Geometry check sheet. Reference: drawing and pictorial views, mm from the part's lowest x, y, z. Give positions to 0.01 mm unless a question says otherwise; leave off trailing zeros. Order: outer loops, then holes, each group sorted by start corner. A loop starts at its lowest first (then second) coordinate and runs counter-clockwise, first axis right, second up.
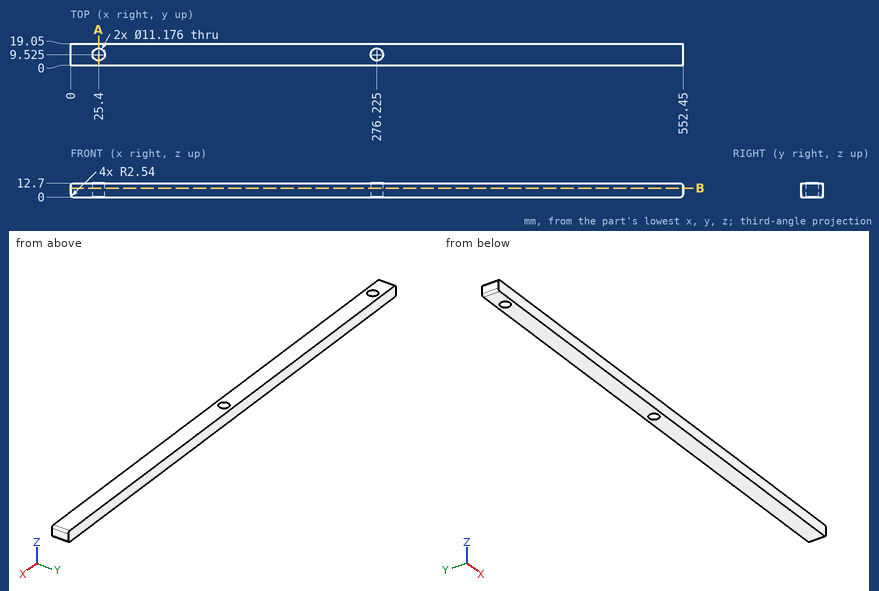
(1) Gauge pin test, flat end, axial feed: pin 1 Ø9 at (x, y) = (25.4, 9.525) entering from -Z. Record the tip position at first contact, or that the pin passes through.
Response values:
pin 1: passes through
(2) Cross-section at B-B on z = 8.25. Enter the section's corners in (x, y) (3 decimals), then the cut area to 3 significant figures.
Response values:
outline: (0, 0) - (552.45, 0) - (552.45, 19.05) - (0, 19.05) - close; hole circle Ø11.176 at (25.4, 9.525); hole circle Ø11.176 at (276.225, 9.525)
area: 10,300 mm2
(3) Cross-section at A-A on x = 25.4. Enter the section's corners in (y, z), then the cut area to 4 significant figures.
Response values:
outline: (0, 0) - (3.94, 0) - (3.94, 12.7) - (0, 12.7) - close; (15.11, 0) - (19.05, 0) - (19.05, 12.7) - (15.11, 12.7) - close
area: 100.0 mm2
(4) Material ranges on L1, parallel to X at y = 9, z = 8; L2, parallel to X at y = 9.75, z = 8.5; L3, parallel to Y at x = 25.4, z = 2.75, recorded low to high.
Response values:
L1: x = 0 to 19.84, 30.96 to 270.66, 281.79 to 552.45
L2: x = 0 to 19.82, 30.98 to 270.64, 281.81 to 552.45
L3: y = 0 to 3.94, 15.11 to 19.05
